Could you check a few things on this drawing? It's one solid part, dimensions in mm from its lowest x, y, z. Coordinates: 2 decimals unless noted, no trailing zeros. Order: outer loops, then holes, each group sorted by start corner. A loop starts at its lowest first (then second) coordinate and runs counter-clockwise, first axis right, second up. Notation, with made-up numbers: (-17, -8.5) - (10, -8.5) arc R19 cw to (10, 5.5) - close; hole circle Ø8 at (18, 4.25). An arc over 180 degrees is marked (long way). Return JSON: item names as keys, results as strings. Group by question number.
1) Imagine slicing it at B-B (z = 19.05). Write out the boundary of the cut face in (x, y) (1 decimal), and give its area (3 significant figures).
2) Imagine slicing it at A-A (x = 117). Write out the boundary of the cut face in (y, z).
3) For pin 1 Ø1 at (y, z) = (178.5, 6) entering from -X; pin 2 Ø5 at (x, z) = (19.5, 13) entering from +Y; pin 3 Ø2 at (x, z) = (118.5, 13.5) entering from +Y (1 decimal); pin 4 Ø6.5 at (y, z) = (53.75, 19.05) entering from +X, each with a flat end and sliding along its axis, tell me the tip position at first contact or that it passes through.
4) If I drill on line 1 along Y through (x, z) = (65, 19) (1 decimal); line 2 along Z through (x, y) = (73, 56.5); line 3 along Y through (x, z) = (16, 25.5) (1 decimal), over which ranges is the centre line in solid material (lowest first)?
5) Imagine slicing it at C-C (z = 4.5). Write out the boundary of the cut face in (x, y), and give its area (3 significant figures).
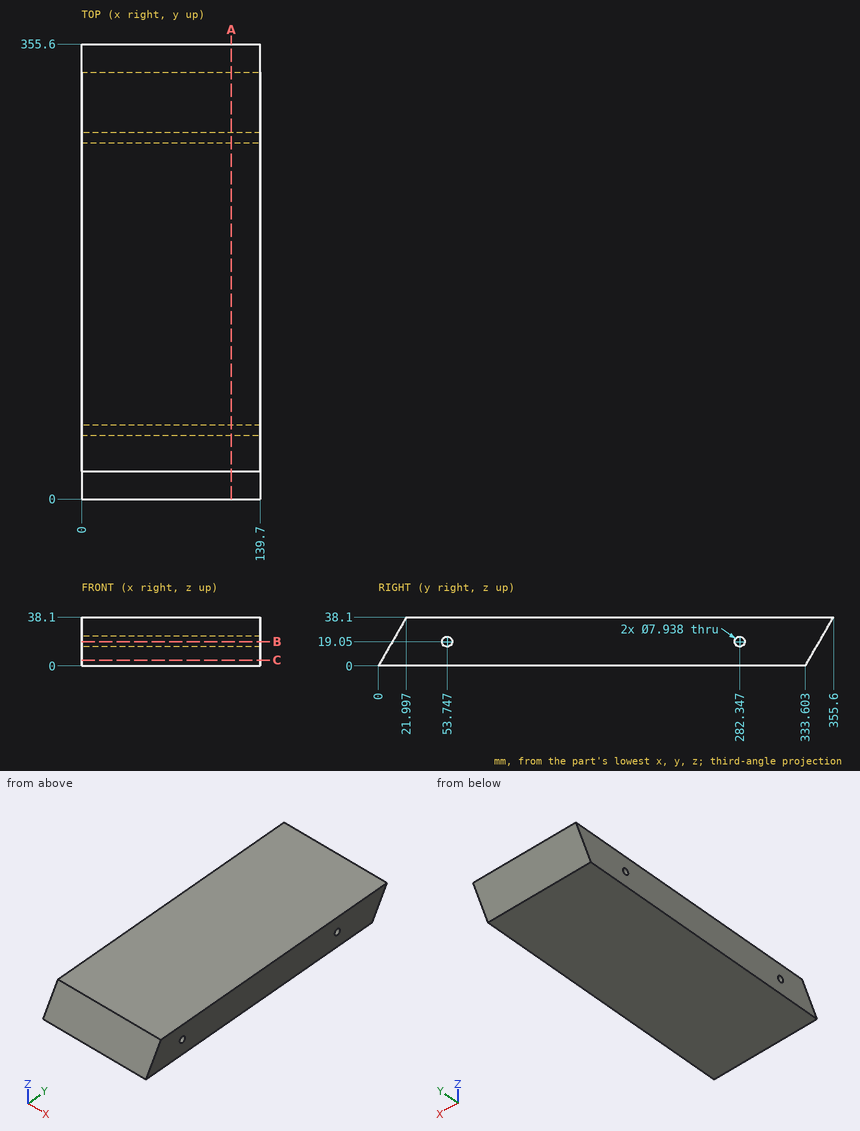
Calculated:
{
 "1": {"outline": "(0, 11) - (139.7, 11) - (139.7, 49.8) - (0, 49.8) - close; (0, 57.7) - (139.7, 57.7) - (139.7, 278.4) - (0, 278.4) - close; (0, 286.3) - (139.7, 286.3) - (139.7, 344.6) - (0, 344.6) - close", "area": "44,400 mm2"},
 "2": {"outline": "(0, 0) - (333.6, 0) - (355.6, 38.1) - (22, 38.1) - close; hole circle Ø7.94 at (53.75, 19.05); hole circle Ø7.94 at (282.35, 19.05)"},
 "3": {"pin 1": "x = 0", "pin 2": "y = 342.55", "pin 3": "y = 342", "pin 4": "through"},
 "4": {"line 1": "11 to 49.8, 57.7 to 278.4, 286.3 to 344.6", "line 2": "0 to 16.19, 21.91 to 38.1", "line 3": "14.7 to 348.3"},
 "5": {"outline": "(0, 2.6) - (139.7, 2.6) - (139.7, 336.2) - (0, 336.2) - close", "area": "46,600 mm2"}
}
